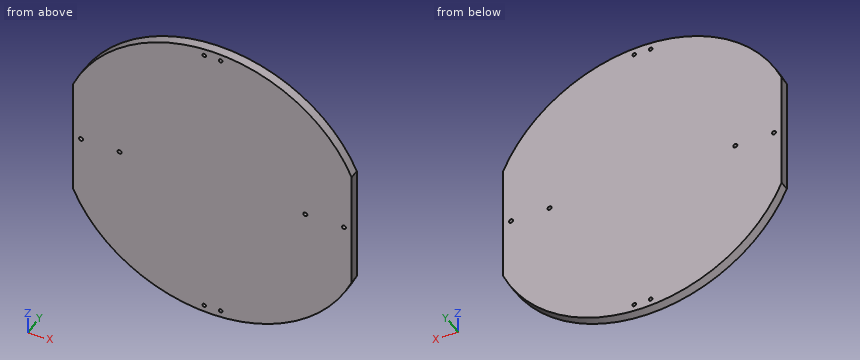
```python
from build123d import *

# Parameters (mm, degrees)
CROQUIS1_R              = 1.65
CROQUIS1_R_2            = 1.5
SALIENTE_EXTRUIR1_DEPTH = 8


with BuildPart() as part:
    # Croquis1 → Saliente-Extruir1 (new body)
    with BuildSketch(Plane(origin=(0, 0, 0), x_dir=(1, 0, 0), z_dir=(0, 1, 0))):
        with BuildLine():
            Line((-114.564392374, -50), (-114.564392374, 50))
            ThreePointArc((-114.564392374, 50), (0, 125), (114.564392374, 50))
            Line((114.564392374, 50), (114.564392374, -50))
            ThreePointArc((114.564392374, -50), (0, -125), (-114.564392374, -50))
        make_face()
        with Locations((108.164392374, 0)):
            Circle(CROQUIS1_R, mode=Mode.SUBTRACT)
        with Locations((76.414392374, 0)):
            Circle(CROQUIS1_R, mode=Mode.SUBTRACT)
        with Locations((-108.164392374, 0)):
            Circle(CROQUIS1_R, mode=Mode.SUBTRACT)
        with Locations((-76.414392374, 0)):
            Circle(CROQUIS1_R, mode=Mode.SUBTRACT)
        with Locations((-6.75, 118.95)):
            Circle(CROQUIS1_R_2, mode=Mode.SUBTRACT)
        with Locations((6.75, 118.95)):
            Circle(CROQUIS1_R_2, mode=Mode.SUBTRACT)
        with Locations((6.75, -118.95)):
            Circle(CROQUIS1_R_2, mode=Mode.SUBTRACT)
        with Locations((-6.75, -118.95)):
            Circle(CROQUIS1_R_2, mode=Mode.SUBTRACT)
    extrude(amount=SALIENTE_EXTRUIR1_DEPTH)


solid = part.part
```
Source: CAD feature listing. Evaluate the final solid. Frame: model axes, mm. Give positions to 0.01 mm unless a question says otherwise; leave off trailing zeros. Loops run counter-clockwise (first coordinate to the right, second up) from the corner with the lowest first, then second, coordinate; pieces in that order, holes last. Notation, with made-up numbers: (45, -23.5) -> (99, -23.5) arc R15 ccw to (99, -7.5) -> close; hole circle Ø10 at (48, 15). An arc over 180 degrees is marked (long way). Put each result on its own line as item: value. Start each with the question number.
1) Cut plane C-C (z = 101.5). Return loops of the section in (x, y).
2) Cut plane A-A (y = 4). State how many separate pieces and enclosed holes the cut face has, then the cut area to 3 significant figures.
3) Contact query for flat-ended pins moving along their axis: P1, Ø5, axis at x = -6.75, z = -118.95, coming from the +Y side; P2, Ø1, axis at x = 16.5, y = 2.5, coming from the -Z side. Output: stop coordinate, or through.
4) Cut plane B-B (x = -50). Return loops of the section in (y, z).
5) Material intervals for probe 1 along X at (y, z) = (5, 0); probe 2 along Z at (x, y) = (-6.75, 3); probe 3 along X at (y, z) = (5.5, -88) (3 decimals), sorted ascending.
Results are:
1. outline: (-72.96, 0) -> (72.96, 0) -> (72.96, 8) -> (-72.96, 8) -> close
2. separate pieces: 1
2. enclosed holes: 8
2. area: 47,600 mm2
3. P1: stops at y = 8
3. P2: stops at z = -123.97
4. outline: (0, -114.56) -> (8, -114.56) -> (8, 114.56) -> (0, 114.56) -> close
5. probe 1: x = -114.56 to -109.81, -106.51 to -78.06, -74.76 to 74.76, 78.06 to 106.51, 109.81 to 114.56
5. probe 2: z = -124.82 to -120.45, -117.45 to 117.45, 120.45 to 124.82
5. probe 3: x = -88.775 to 88.775
